from build123d import *

# Parameters (mm, degrees)
DODANIE_WYCI_GNI_CIE1_DEPTH = 10
SZKIC3_W                    = 10
SZKIC3_H                    = 10
DODANIE_WYCI_GNI_CIE2_DEPTH = 1
ZAOKR_GLENIE1_R             = 3
ZAOKR_GLENIE2_R             = 3
SZKIC5_R                    = 2.5
WYTNIJ_WYCI_GNI_CIE1_DEPTH  = 1
ZAOKR_GLENIE1_OF_LUSTRO1_R  = 3
ZAOKR_GLENIE2_OF_LUSTRO1_R  = 3


with BuildPart() as part:
    # Szkic2 → Dodanie-wyciągnięcie1 (new body)
    with BuildSketch(Plane(origin=(0, 0, 0), x_dir=(1, 0, 0), z_dir=(0, 1, 0))):
        with BuildLine():
            Line((-43, 43), (-42, 43))
            Line((-42, 43), (-42, 0))
            ThreePointArc((-42, 0), (0, -42), (42, 0))
            Line((42, 0), (42, 43))
            Line((42, 43), (43, 43))
            Line((43, 43), (43, 0))
            ThreePointArc((43, 0), (0, -43), (-43, 0))
            Line((-43, 0), (-43, 43))
        make_face()
    extrude(amount=DODANIE_WYCI_GNI_CIE1_DEPTH)

    # Szkic3 → Dodanie-wyciągnięcie2 (add)
    with BuildSketch(Plane(origin=(0, 0, -43), x_dir=(-1, 0, 0), z_dir=(0, 0, -1))):
        with Locations((-48, 5)):
            Rectangle(SZKIC3_W, SZKIC3_H)
    dodanie_wyci_gni_cie2 = extrude(amount=-DODANIE_WYCI_GNI_CIE2_DEPTH)

    # Zaokrąglenie1
    zaokr_glenie1_edges = [part.edges().sort_by_distance(p)[0] for p in [
        (53, 10, -42.5),
    ]]
    fillet(zaokr_glenie1_edges, radius=ZAOKR_GLENIE1_R)

    # Zaokrąglenie2
    zaokr_glenie2_edges = [part.edges().sort_by_distance(p)[0] for p in [
        (53, 0, -42.5),
    ]]
    fillet(zaokr_glenie2_edges, radius=ZAOKR_GLENIE2_R)

    # Szkic5 → Wytnij-wyciągnięcie1 (cut)
    with BuildSketch(Plane(origin=(0, 0, -43), x_dir=(-1, 0, 0), z_dir=(0, 0, -1))):
        with Locations((-48, 5)):
            Circle(SZKIC5_R)
    wytnij_wyci_gni_cie1 = extrude(amount=-WYTNIJ_WYCI_GNI_CIE1_DEPTH, mode=Mode.SUBTRACT)

    # Lustro1: Dodanie-wyciągnięcie2, Wytnij-wyciągnięcie1 across plane
    add(dodanie_wyci_gni_cie2.mirror(Plane(origin=(0, 0, 0), x_dir=(0, 0, 1), z_dir=(1, 0, 0))))
    add(wytnij_wyci_gni_cie1.mirror(Plane(origin=(0, 0, 0), x_dir=(0, 0, 1), z_dir=(1, 0, 0))), mode=Mode.SUBTRACT)

    # Zaokrąglenie1 of Lustro1
    zaokr_glenie1_of_lustro1_edges = [part.edges().sort_by_distance(p)[0] for p in [
        (-53, 10, -42.5),
    ]]
    fillet(zaokr_glenie1_of_lustro1_edges, radius=ZAOKR_GLENIE1_OF_LUSTRO1_R)

    # Zaokrąglenie2 of Lustro1
    zaokr_glenie2_of_lustro1_edges = [part.edges().sort_by_distance(p)[0] for p in [
        (-53, 0, -42.5),
    ]]
    fillet(zaokr_glenie2_of_lustro1_edges, radius=ZAOKR_GLENIE2_OF_LUSTRO1_R)


solid = part.part
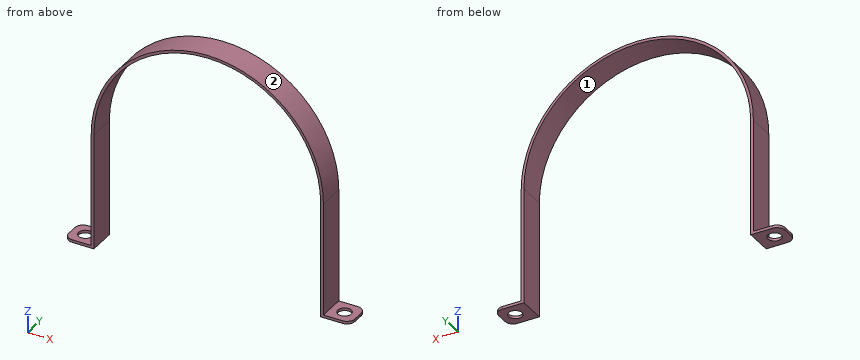
Can you work these out from the model? Positions are in its coordinate system, mm. Face numbers are marked on the shaded views. Coordinates: 2 decimals unless noted, no trailing zeros. Loops run counter-clockwise (first coordinate to the right, second up) from the corner with the lowest first, then second, coordinate; pieces in that order, holes last. Notation, with made-up numbers: (70, 1.5) - (124, 1.5) arc R18 ccw to (124, 7.5) - close; hole circle Ø8 at (82, 42). An arc over 180 degrees is marked (long way). Answer as a JSON object with one key per item and string values. Group by question number.
Item 1: If we section it at C-C (x = 48): List the corners of the cut face in (y, z) for me, plus the area to 3 significant figures.
Item 2: If we mould it in two halves opening along X, with no side actions, what happens to the marked faces 1 and 2? For each: released by +X, released by -X, zero draft, split by the parting line, or undercut.
Item 3: For pin 1 (1 mm diameter, centred on y = 8, z = -27.5, fed in from -X); pin 2 (3 mm diameter, centred on x = 48, y = 5, fed in from -Z); pin 3 (3 mm diameter, centred on y = 6, z = -21.5, fed in from +X); pin 4 (5 mm diameter, centred on y = 8, z = 32.5, fed in from +X), each with a flat end and sliding along its axis, tell me the tip position at first contact or that it passes through.
Item 4: If I drill on L1, parallel to Y at x = 48, z = -42.5; L2, parallel to X at y = 3.25, z = -15.5; L3, parallel to X at y = 8.5, z = 37, over which ranges is the centre line in solid material (lowest first)? Write a range as from..to.
Item 5: If we section it at D-D (x = 0): List the corners of the cut face in (y, z) for me.
Item 6: If we section it at A-A (z = 18): List the corners of the cut face in (x, y) for me, plus the area to 3 significant figures.
Item 7: If we section it at B-B (y = 5): List the corners of the cut face in (x, z) for me, plus the area to 3 significant figures.
Returned:
{
 "1": {"outline": "(0, -43) - (2.5, -43) - (2.5, -42) - (0, -42) - close; (7.5, -43) - (10, -43) - (10, -42) - (7.5, -42) - close", "area": "5.00 mm²"},
 "2": {"face 1": "undercut", "face 2": "split by the parting line"},
 "3": {"pin 1": "stops at x = -43", "pin 2": "passes through", "pin 3": "stops at x = 43", "pin 4": "stops at x = 30.81"},
 "4": {"L1": "y = 0..2.5, 7.5..10", "L2": "x = -43..-42, 42..43", "L3": "x = -21.91..-19.87, 19.87..21.91"},
 "5": {"outline": "(0, 42) - (10, 42) - (10, 43) - (0, 43) - close"},
 "6": {"outline": "(-39.05, 0) - (-37.95, 0) - (-37.95, 10) - (-39.05, 10) - close; (37.95, 0) - (39.05, 0) - (39.05, 10) - (37.95, 10) - close", "area": "22.1 mm²"},
 "7": {"outline": "(-53, -43) - (-50.5, -43) - (-50.5, -42) - (-53, -42) - close; (-45.5, -43) - (-42, -43) - (-42, 0) arc R42 cw to (42, 0) - (42, -43) - (45.5, -43) - (45.5, -42) - (43, -42) - (43, 0) arc R43 ccw to (-43, 0) - (-43, -42) - (-45.5, -42) - close; (50.5, -43) - (53, -43) - (53, -42) - (50.5, -42) - close", "area": "230 mm²"}
}
